Autodesk Fusion 360 part; units mm, degrees
sketch "Sketch1" plane through (0, 0, 0) normal (0, 0, 1) x (1, 0, 0)
  line L0 (0, 0) -> (15, 0)
  line L1 (15, 0) -> (15, 20)
  line L2 (15, 20) -> (0, 20)
  line L3 (0, 20) -> (0, 0)
  line L4 (0, 20) -> (-30, 20)
  line L5 (15, 20) -> (45, 20)
  line L6 (45, 20) -> (28.4651, 45.8146)
  line L7 (28.4651, 45.8146) -> (39.0949, 45.8146)
  line L8 (39.0949, 45.8146) -> (20.1808, 77.3096)
  line L9 (20.1808, 77.3096) -> (28.3002, 77.3096)
  line L10 (28.3002, 77.3096) -> (7.5, 108.6082)
  line L11 (-13.3002, 77.3096) -> (7.5, 108.6082)
  line L12 (-5.1808, 77.3096) -> (-13.3002, 77.3096)
  line L13 (-24.0949, 45.8146) -> (-5.1808, 77.3096)
  line L14 (-13.4651, 45.8146) -> (-24.0949, 45.8146)
  line L15 (-30, 20) -> (-13.4651, 45.8146)
  dimension "d1" = 15
  dimension "d2" = 20
  dimension "d3" = 30
extrude "Extrude1" add sketch "Sketch1" along normal blind 10 contours L2 L4 L5 L6 L7 L8 L9 L10 L11 L12 L13 L14 L15
extrude "Extrude2" add sketch "Sketch1" along normal blind 7 contours L0 L1 L2 L3
sketch "Sketch2" plane through (0, 0, 10) normal (0, 0, 1) x (-1, 0, 0)
  line L0 (30, -20) -> (-45, -20)
  line L1 (-45, -20) -> (-28.4651, -45.8146)
  line L2 (-28.4651, -45.8146) -> (-39.0949, -45.8146)
  line L3 (-39.0949, -45.8146) -> (-20.1808, -77.3096)
  line L4 (-20.1808, -77.3096) -> (-28.3002, -77.3096)
  line L5 (-28.3002, -77.3096) -> (-7.5, -108.6082)
  line L6 (-7.5, -108.6082) -> (13.3002, -77.3096)
  line L7 (13.3002, -77.3096) -> (5.1808, -77.3096)
  line L8 (5.1808, -77.3096) -> (24.0949, -45.8146)
  line L9 (24.0949, -45.8146) -> (13.4651, -45.8146)
  line L10 (13.4651, -45.8146) -> (30, -20)
  circle A0 centre (6.0624, -88.2005) radius 2.5
  circle A1 centre (-24.9742, -69.3278) radius 3.5
  circle A2 centre (-0.4251, -41.565) radius 3
  circle A3 centre (-25.1078, -32.9073) radius 3.5
  circle A4 centre (-13.8678, -88.9006) radius 3
  circle A5 centre (12.6203, -64.9216) radius 4
  circle A6 centre (-4.4215, -78.0323) radius 2.5
  circle A7 centre (-11.665, -58.7996) radius 4
  circle A8 centre (-7.5, -108.6082) radius 4
  circle A9 centre (14.6379, -30.0753) radius 2.5
  circle A10 centre (-35.8887, -51.1535) radius 3
  dimension "d8" = 5
  dimension "d9" = 7
  dimension "d10" = 6
  dimension "d11" = 7
  dimension "d12" = 6
  dimension "d13" = 8
  dimension "d14" = 5
  dimension "d15" = 8
  dimension "d16" = 8
  dimension "d17" = 5
  dimension "d18" = 6
extrude "Extrude3" add sketch "Sketch2" along normal blind 3 contours L3 A1 | L3 A1 | L5 L6 A8 | L5 L6 A8 | A2 | A6
extrude "Extrude4" add sketch "Sketch2" along normal blind 2 contours L6 A0 | L6 A0 | A4 | A9
extrude "Extrude5" add sketch "Sketch2" along normal blind 1 contours L8 A5 | L8 A5 | L3 A10 | L3 A10 | A3 | A7
extrude "Extrude6" add sketch "Sketch2" against normal blind 10 contours L8 A5 | L3 A10 | L3 A1 | L6 A0 | L5 L6 A8 picked at (11.992, -63.5572) picked at (-37.2683, -51.7586) picked at (-26.1307, -69.1738) picked at (5.2322, -88.2727) picked at (-8.8058, -106.2913)
sketch "Sketch3" plane through (0, 0, 0) normal (0, 0, 1) x (1, 0, 0)
  line L0 (45, 20) -> (15, 20)
  line L1 (15, 20) -> (15, 0)
  line L2 (15, 0) -> (0, 0)
  line L3 (0, 0) -> (0, 20)
  line L4 (0, 20) -> (-30, 20)
  line L5 (-30, 20) -> (-13.4651, 45.8146)
  line L6 (-13.4651, 45.8146) -> (-24.0949, 45.8146)
  line L7 (-24.0949, 45.8146) -> (-14.6797, 61.4925)
  arc A0 (-10.561, 68.3508) -> (-14.6797, 61.4925) centre (-12.6203, 64.9216) ccw
  line L8 (-10.561, 68.3508) -> (-5.1808, 77.3096)
  line L9 (-5.1808, 77.3096) -> (-13.3002, 77.3096)
  line L10 (-13.3002, 77.3096) -> (-7.4461, 86.1184)
  arc A1 (-4.6787, 90.2827) -> (-7.4461, 86.1184) centre (-6.0624, 88.2005) ccw
  line L11 (-4.6787, 90.2827) -> (5.286, 105.2768)
  arc A2 (9.714, 105.2768) -> (5.286, 105.2768) centre (7.5, 108.6082) ccw
  line L12 (9.714, 105.2768) -> (28.3002, 77.3096)
  line L13 (28.3002, 77.3096) -> (20.1808, 77.3096)
  line L14 (20.1808, 77.3096) -> (23.1723, 72.3283)
  arc A3 (26.7762, 66.3273) -> (23.1723, 72.3283) centre (24.9742, 69.3278) ccw
  line L15 (26.7762, 66.3273) -> (34.3442, 53.7254)
  arc A4 (37.4332, 48.5817) -> (34.3442, 53.7254) centre (35.8887, 51.1535) ccw
  line L16 (37.4332, 48.5817) -> (39.0949, 45.8146)
  line L17 (39.0949, 45.8146) -> (28.4651, 45.8146)
  line L18 (28.4651, 45.8146) -> (45, 20)
  circle A5 centre (4.4215, 78.0323) radius 2.5
  circle A6 centre (-12.6203, 64.9216) radius 4
  line L19 (7.5, 108.6082) -> (-13.3002, 77.3096)
  circle A7 centre (-6.0624, 88.2005) radius 2.5
  circle A8 centre (13.8678, 88.9006) radius 3
  circle A9 centre (7.5, 108.6082) radius 4
  circle A10 centre (24.9742, 69.3278) radius 3.5
  circle A11 centre (24.9742, 69.3278) radius 3.5
  circle A12 centre (11.665, 58.7996) radius 4
  circle A13 centre (0.4251, 41.565) radius 3
  circle A14 centre (25.1078, 32.9073) radius 3.5
  circle A15 centre (-14.6379, 30.0753) radius 2.5
  circle A16 centre (35.8887, 51.1535) radius 3
  line L20 (0, 20) -> (0, 0)
  line L21 (0, 0) -> (15, 0)
  line L22 (15, 0) -> (15, 20)
  line L23 (15, 20) -> (0, 20)
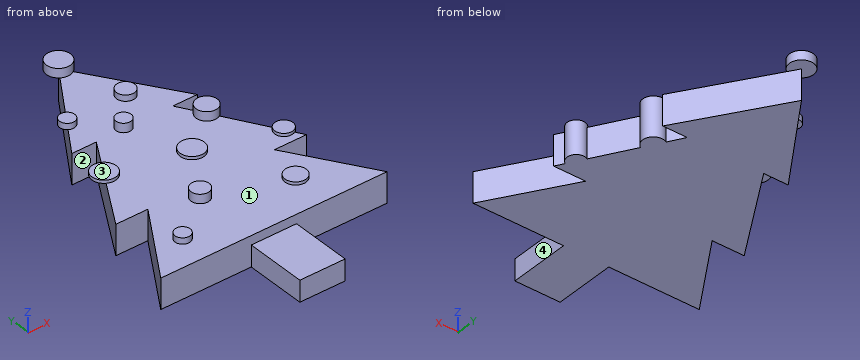
Here's how the part is built. I have some questions about the finished solid (model axes, mm). Face numbers are marked on the shaded views. A direction names the side the tool comes from. Coordinates: 2 decimals unless noted, no trailing zeros. Order: outer loops, then holes, each group sorted by start corner. A loop starts at its lowest first (then second) coordinate and runs counter-clockwise, first axis right, second up.
Item 1: If we section it at A-A, the plane z = 5: List the corners of the cut face in (x, y) for me.
Response values:
outline: (-30, 20) - (0, 20) - (0, 0) - (15, 0) - (15, 20) - (45, 20) - (28.47, 45.81) - (39.09, 45.81) - (37.43, 48.58) arc R3 ccw to (34.34, 53.73) - (26.78, 66.33) arc R3.5 ccw to (23.17, 72.33) - (20.18, 77.31) - (28.3, 77.31) - (7.5, 108.61) - (-13.3, 77.31) - (-5.18, 77.31) - (-24.09, 45.81) - (-13.47, 45.81) - close
Item 2: I'm going to push flat-ended pins straight in: pin 1 Ø9 at (x, y) = (-12.5, 66) entering from +Z; pin 2 Ø3 at (x, z) = (32.5, 5.5) entering from -Y; pin 3 Ø5 at (x, y) = (14, 89.5) entering from +Z; pin 4 Ø3 at (x, y) = (-13, 66.5) entering from -Z. Where does each tip first touch, or does it pass through?
Response values:
pin 1: stops at z = 11
pin 2: stops at y = 20
pin 3: stops at z = 12
pin 4: stops at z = 0
Item 3: I need wall thicknesses on probe 1 along Y at (x, z) = (39.5, 6); probe 2 along X at (y, z) = (15, 2.25); probe 3 along Y at (x, z) = (23.5, 4.5). Which ranges of each line are inside material? Lowest first, please.
Response values:
probe 1: y = 20 to 28.59
probe 2: x = 0 to 15
probe 3: y = 20 to 72.5, 77.31 to 84.53
Item 4: Which directions (+Z, -Z, +X, -X, +Y, -Y) give clear straight access to the entire face, cutting with the end or side of a thin tool? Please do the marked faces 1, 2, 3 and 4.
Response values:
face 1: +Z
face 2: +Z, -Z, -X
face 3: +Z, -X, +Y
face 4: +Z, -Z, +X, -Y
